Model file for the job. Use its own axes, mm. A direction names the side the tool comes from. Round coordinates to 2 decimals unless told otherwise and drop trailing zeros. Loops run counter-clockwise (first coordinate to the right, second up) from the corner with the lowest first, then second, coordinate; pieces in that order, holes last. Notation, with made-up numbers: M -27.5,-31 L 6.5,-31 A18 ccw 6.5,-7 Z; hole C -23,16.25 d11. An arc over 180 degrees is marked long. Use a Markdown table: item, result. Add a question column.
Q1. Pin check, flat tips, straight feed: pin 1 (5 mm diameter, centred on y = 59.5, z = 6.5, fed in from -X); pin 2 (14 mm diameter, centred on x = 19.5, z = 3, fed in from +Y); pin 3 (12 mm diameter, centred on y = 21.5, z = -11, fed in from +X). Stop position of each tip, or through.
Q2. Tool access for faces 5 (the face through (25, 6.35, 0)), 6 (the face through (3.13, 23.21, 0.18)): list every direction of +Z, -Z, +X, -X, +Y, -Y with a clear straight run to the whole face (end or side of a thin tool).
Q3. Mould opens along X. For faces 1 (the face through (3.131, 53.302, -1.595)), 2 (the face through (0, 38, 0)), 3 (the face through (36.29, 4.44, 0.23)), 4 (the face through (23.023, 3.131, 1.251)) say: +X half, -X half, draft (parallel to the pull), parting line (faces both ways), or undercut.
Q4. Cut at D-D (y = 47). Give the cut face in (x, z), plus the area to 3 significant figures.
Q5. Cut at C-C (z = 1.5). State how many separate pieces and enclosed holes the cut face has, plus the area to 3 significant figures.
Q6. Cut at A-A (y = 19.05). Give the cut face in (x, z).
Q7. Probe line 1 (Z direction, x = 1.5, y = 57.15); line 2 (Y direction, x = 14, z = 8.5). List the from-to ranges inside material, lowest first. Write a range as from..to.
from build123d import *

# Parameters (mm, degrees)
BOSS_EXTRUDE1_DEPTH = 16.637
FILLET1_R           = 6.35
SKETCH3_R           = 4.1656
CUT_EXTRUDE1_DEPTH  = 87.803454822
SKETCH4_R           = 4.1656
CUT_EXTRUDE2_DEPTH  = 87.803454822


with BuildPart() as part:
    # Sketch2 → Boss-Extrude1 (new, symmetric)
    with BuildSketch(Plane.XY):
        with BuildLine():
            Line((0, 0), (0, 76.2))
            Line((0, 76.2), (6.35, 76.2))
            Line((6.35, 76.2), (6.35, 14.2748))
            ThreePointArc((6.35, 14.2748), (8.67112018, 8.67112018), (14.2748, 6.35))
            Line((14.2748, 6.35), (38.1, 6.35))
            Line((38.1, 6.35), (38.1, 0))
            Line((38.1, 0), (0, 0))
        make_face()
    extrude(amount=BOSS_EXTRUDE1_DEPTH, both=True)

    # Fillet1
    fillet1_edges = [part.edges().sort_by_distance(p)[0] for p in [
        (38.1, 6.35, 0),
        (6.35, 76.2, 0),
    ]]
    fillet(fillet1_edges, radius=FILLET1_R - 0.0001)  # a hair under: the kernel refuses the full size

    # Sketch3 → Cut-Extrude1 (cut, through all)
    with BuildSketch(Plane.ZY):
        with Locations(Location((0, 57.15, 0), (0, 0, 270))):
            Circle(SKETCH3_R)
        with Locations(Location((0, 19.05, 0), (0, 0, 270))):
            Circle(SKETCH3_R)
    extrude(amount=-CUT_EXTRUDE1_DEPTH, mode=Mode.SUBTRACT)

    # Sketch4 → Cut-Extrude2 (cut, through all)
    with BuildSketch(Plane.XZ):
        with Locations((19.05, 0)):
            Circle(SKETCH4_R)
    extrude(amount=-CUT_EXTRUDE2_DEPTH, mode=Mode.SUBTRACT)


solid = part.part
Checked values:
| question | item | result |
|---|---|---|
| 1 | pin 1 | stops at x = 0 |
| 1 | pin 2 | stops at y = 6.55 |
| 1 | pin 3 | stops at x = 6.35 |
| 2 | face 5 | +Z, -Z, +X, +Y |
| 2 | face 6 | +X, -X |
| 3 | face 1 | draft |
| 3 | face 2 | -X half |
| 3 | face 3 | +X half |
| 3 | face 4 | undercut |
| 4 | outline | M 0,-16.64 L 6.35,-16.64 L 6.35,16.64 L 0,16.64 Z |
| 4 | area | 211 mm^2 |
| 5 | separate pieces | 4 |
| 5 | enclosed holes | 0 |
| 5 | area | 534 mm^2 |
| 6 | outline | M 0,-16.64 L 6.35,-16.64 L 6.35,-4.17 L 0,-4.17 Z; M 0,4.17 L 6.35,4.17 L 6.35,16.64 L 0,16.64 Z |
| 7 | line 1 | z = -16.64..-4.17, 4.17..16.64 |
| 7 | line 2 | y = 0..6.35 |
